CAD build for the part. Positions are in the model's coordinates, mm. A direction names the side the tool comes from. Coordinates: 2 decimals unless noted, no trailing zeros. Write each loop counter-clockwise with the first axis right and the second up, starting at its lowest first coordinate (ties: lowest second). Pieces come first, ordered by that corner, then holes. Notation, with made-up numbers: (-26.75, 4) - (-13.75, 4) arc R17 cw to (-13.75, 30) - close; hole circle Ø11 at (-8, 53). An arc over 180 degrees is marked (long way). Answer in a Markdown table with one row per item. Add a question column.
Q1. Band-saw the part on A-A (x = 0). List the corners of the cut face in (y, z), and give its area (3 significant figures).
Q2. Pin check, flat tips, straight feed: pin 1 (8 mm diameter, centred on x = -16, z = 4.5, fed in from -Y); pin 2 (1 mm diameter, centred on y = 27, z = 17.5, fed in from -X); pin 3 (10 mm diameter, centred on y = 8.5, z = 3.5, fed in from +X). Stop position of each tip, or through.
Q3. Band-saw the part on D-D (x = -8.5). List the corners of the cut face in (y, z).
Q4. Band-saw the part on C-C (z = 18.25). State how many separate pieces and enclosed holes the cut face has, and give its area (3 significant figures).
Q5. 3-axis set-ups, long thin cutter, end or side, ignore diameter. For faces 4 (the cylindrical face through (-0.83, 59.41, 8.38)), 5 (the flat face through (0, 120, 6)), 6 (the flat face through (0, 61, 0)): which of +Z, -Z, +X, -X, +Y, -Y reach the whole face in a straight line?
Q6. Two-plate mould, pull along X, no slides. Class faces 1 (the cylindrical face through (3.902, -17.572, 13.395)), 2 (the flat face through (0, 61, 21)), 3 (the flat face through (0, 0, 6)): +X half, -X half, draft (parallel to the pull), parting line (faces both ways), or undercut.
Q7. Drill centre lines: line 1 along Y through (x, z) = (0, 18.25); line 2 along Y through (x, z) = (6.5, 13); line 3 along Y through (x, z) = (0, 12.25). Where is each one in solid material? Low to high. Write a range as from..to.
Q8. Band-saw the part on B-B (y = 120). List the corners of the cut face in (x, z), and give its area (3 significant figures).
```python
from build123d import *

# Parameters (mm, degrees)
SKETCH1_R             = 21
BOSS_EXTRUDE2_DEPTH   = 5
BOSS_EXTRUDE2_2_DEPTH = 5
BOSS_EXTRUDE5_DEPTH   = 16
SKETCH8_R             = 18
CUT_EXTRUDE3_DEPTH    = 144.342247908
BOSS_EXTRUDE6_START   = 5
BOSS_EXTRUDE6_DEPTH   = 5
SKETCH10_R            = 2.75
CUT_EXTRUDE4_DEPTH    = 114


with BuildPart() as part:
    # Sketch1 → Boss-Extrude2 (new body)
    with BuildSketch(Plane.XY):
        with Locations((0, 120)):
            Circle(SKETCH1_R)
    extrude(amount=BOSS_EXTRUDE2_DEPTH)



with BuildPart() as body_2:
    # Sketch1 → Boss-Extrude2 2 (new body)
    with BuildSketch(Plane.XY):
        Circle(SKETCH1_R)
    extrude(amount=BOSS_EXTRUDE2_2_DEPTH)


with BuildPart() as part_1:
    add(part.part)

    add(body_2.part)  # Boss-Extrude5 merges body 2
    # Sketch5 → Boss-Extrude5 (add)
    with BuildSketch(Plane.XY.offset(5)):
        with BuildLine():
            add(Edge.make_bspline(
                [(-20.124611797, 114), (-17.072662318, 103.763450251), (-12.954200117, 66.897613413), (-14.18067636, 25.936565539), (-20.124611797, 6)],
                knots=[0, 0, 0, 0, 0.316724685, 1, 1, 1, 1], degree=3))
            ThreePointArc((-20.124611797, 6), (0, -21), (20.124611797, 6))
            add(Edge.make_bspline(
                [(20.124611797, 114), (17.072662318, 103.763450251), (12.954200117, 66.897613413), (14.18067636, 25.936565539), (20.124611797, 6)],
                knots=[0, 0, 0, 0, 0.316724685, 1, 1, 1, 1], degree=3))
            ThreePointArc((20.124611797, 114), (0, 141), (-20.124611797, 114))
        make_face()
    extrude(amount=BOSS_EXTRUDE5_DEPTH)

    # Sketch8 → Cut-Extrude3 (cut, through all)
    with BuildSketch(Plane(origin=(0, 0, 6), x_dir=(-1, 0, 0), z_dir=(0, 0, -1))):
        with Locations((0, 120)):
            Circle(SKETCH8_R)
        Circle(SKETCH8_R)
    extrude(amount=-CUT_EXTRUDE3_DEPTH, mode=Mode.SUBTRACT)

    # Sketch9 → Boss-Extrude6 (add)
    with BuildSketch(Plane(origin=(0, 0, 5), x_dir=(-1, 0, 0), z_dir=(0, 0, -1)).offset(BOSS_EXTRUDE6_START)):
        with BuildLine():
            ThreePointArc((-20.124611797, 114), (0, 99), (20.124611797, 114))
            add(Edge.make_bspline(
                [(20.124611797, 6), (14.18067636, 25.936565539), (12.954200117, 66.897613413), (17.072662318, 103.763450251), (20.124611797, 114)],
                knots=[0, 0, 0, 0, 0.683275315, 1, 1, 1, 1], degree=3))
            ThreePointArc((20.124611797, 6), (0, 21), (-20.124611797, 6))
            add(Edge.make_bspline(
                [(-20.124611797, 114), (-17.072662318, 103.763450251), (-12.954200117, 66.897613413), (-14.18067636, 25.936565539), (-20.124611797, 6)],
                knots=[0, 0, 0, 0, 0.316724685, 1, 1, 1, 1], degree=3))
        make_face()
    extrude(amount=-BOSS_EXTRUDE6_DEPTH)

    # Sketch10 → Cut-Extrude4 (cut)
    with BuildSketch(Plane(origin=(0, 0, 0), x_dir=(1, 0, 0), z_dir=(0, 1, 0))):
        with Locations(Location((0, -11, 0), (0, 0, 90))):
            Circle(SKETCH10_R)
    extrude(amount=CUT_EXTRUDE4_DEPTH, mode=Mode.SUBTRACT)


solid = part_1.part
```
Checked values:
| question | item | result |
|---|---|---|
| 1 | outline | (-21, 0) - (141, 0) - (141, 21) - (138, 21) - (138, 6) - (102, 6) - (102, 8.25) - (18, 8.25) - (18, 6) - (-18, 6) - (-18, 21) - (-21, 21) - close; (18, 13.75) - (102, 13.75) - (102, 21) - (18, 21) - close |
| 1 | area | 1,860 mm² |
| 2 | pin 1 | stops at y = -17.23 |
| 2 | pin 2 | stops at x = -16 |
| 2 | pin 3 | stops at x = 20.71 |
| 3 | outline | (-19.2, 0) - (139.2, 0) - (139.2, 21) - (135.87, 21) - (135.87, 6) - (104.13, 6) - (104.13, 21) - (15.87, 21) - (15.87, 6) - (-15.87, 6) - (-15.87, 21) - (-19.2, 21) - close |
| 4 | separate pieces | 1 |
| 4 | enclosed holes | 2 |
| 4 | area | 3,300 mm² |
| 5 | face 4 | none |
| 5 | face 5 | +Z |
| 5 | face 6 | -Z, +X, -X, +Y, -Y |
| 6 | face 1 | undercut |
| 6 | face 2 | draft |
| 6 | face 3 | undercut |
| 7 | line 1 | y = -21..-18, 18..102, 138..141 |
| 7 | line 2 | y = -19.97..-16.79, 16.79..103.21, 136.79..139.97 |
| 7 | line 3 | y = -21..-18, 138..141 |
| 8 | outline | (-21, 0) - (21, 0) - (21, 21) - (18, 21) - (18, 6) - (-18, 6) - (-18, 21) - (-21, 21) - close |
| 8 | area | 342 mm² |
